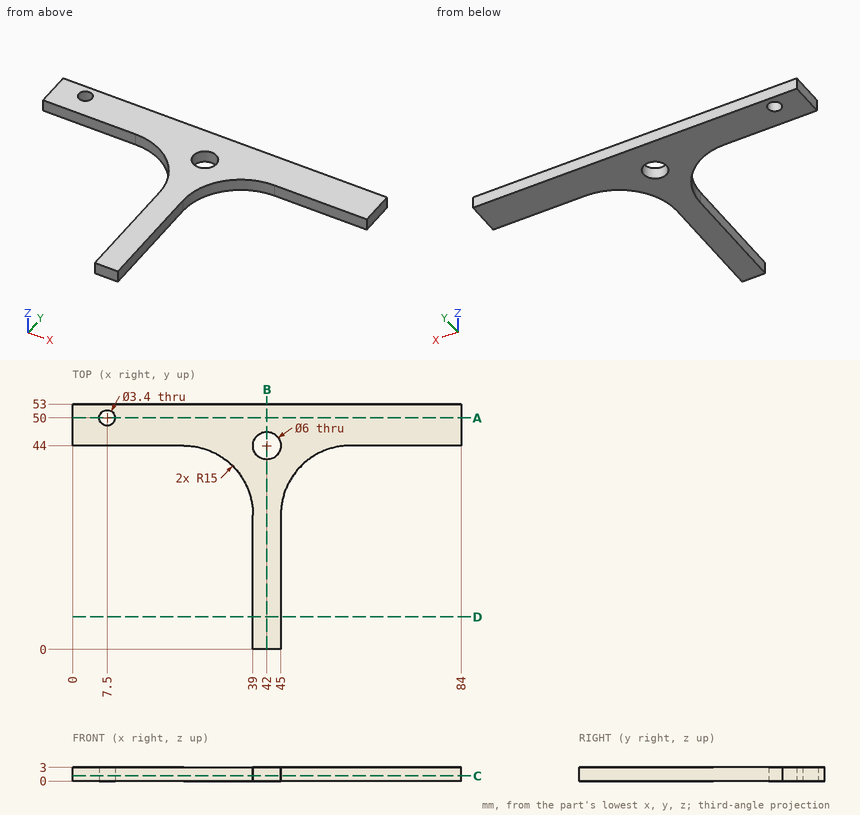
The figure shows three views and two pictorial views of one solid part (mm, origin at its lowest corner). Answer the questions. Round coordinates to 2 decimals unless told otherwise and drop trailing zeros. Loops run counter-clockwise (first coordinate to the right, second up) from the corner with the lowest first, then second, coordinate; pieces in that order, holes last. Notation, with made-up numbers: M 59.25,23.25 L 99.25,23.25 A23 cw 99.25,51.25 Z; hole C 76.5,77.25 d10. An arc over 180 degrees is marked long. Return JSON: item names as keys, results as strings.
Q1. Find section D-D, the plane y = 7. Determine the outline of the cut face in (x, z).
Results list:
{"outline": "M 39,0 L 45,0 L 45,3 L 39,3 Z"}
Q2. Find section B-B, the plane x = 42. Determine the outline of the cut face in (y, z), plus the area to 3 significant figures.
Results list:
{"outline": "M 0,0 L 41,0 L 41,3 L 0,3 Z; M 47,0 L 53,0 L 53,3 L 47,3 Z", "area": "141 mm2"}
Q3. Find section A-A, the plane y = 50. Determine the outline of the cut face in (x, z).
Results list:
{"outline": "M 0,0 L 5.8,0 L 5.8,3 L 0,3 Z; M 9.2,0 L 84,0 L 84,3 L 9.2,3 Z"}
Q4. This flat-tipped pin is pushed along its axis until it touches: pin 1 Ø3.5 at (x, y) = (42, 44) entering from +Z. Where does it stop, or does it pass through?
Results list:
{"pin 1": "passes through"}
Q5. Find the intervals of material crossed by line 1 along Y through (x, z) = (42, 2.3); line 2 along X through (y, z) = (50, 1.2); line 3 along Y through (x, z) = (61.5, 2.3), in increasing order. Write a range as from..to.
Results list:
{"line 1": "y = 0..41, 47..53", "line 2": "x = 0..5.8, 9.2..84", "line 3": "y = 44..53"}
Q6. Find section C-C, the plane z = 1.15. Determine the outline of the cut face in (x, y).
Results list:
{"outline": "M 0,44 L 24,44 A15 cw 39,29 L 39,0 L 45,0 L 45,29 A15 cw 60,44 L 84,44 L 84,53 L 0,53 Z; hole C 7.5,50 d3.4; hole C 42,44 d6"}
